```python
from build123d import *

# Parameters (mm, degrees)
BROCA_DE_ROSQUEAR_PARA_TARRAXA_DE_M51_D     = 4.2
BROCA_DE_ROSQUEAR_PARA_TARRAXA_DE_M51_DEPTH = 10
BROCA_DE_ROSQUEAR_PARA_TARRAXA_DE_M51_TIP   = 1.2618073
CORTE_EXTRUS_O1_DEPTH                       = 69.373971656
CORTE_EXTRUS_O1_DEPTH_BACK                  = 69.373971656
ESBO_O8_W                                   = 1
ESBO_O8_H                                   = 4


with BuildPart() as part:
    # Esboço1 → Revolução1 (revolve)
    with BuildSketch(Plane.XY, mode=Mode.PRIVATE) as revolu_o1_sk:
        Polygon((0, 0), (-5, 0), (-5, 60), (-15, 60), (-15, 65), (0, 65), align=None)
    revolve(revolu_o1_sk.sketch.rotate(Axis((0, 0, 0), (0, 1, 0)), 270), axis=Axis((0, 0, 0), (0, 1, 0)))

    # Broca de rosquear para tarraxa de M51
    with Locations(Plane(origin=(0, 0, 0), x_dir=(-1, 0, 0), z_dir=(0, -1, 0))):
        with Locations((0, 0)):
            Hole(BROCA_DE_ROSQUEAR_PARA_TARRAXA_DE_M51_D / 2, depth=BROCA_DE_ROSQUEAR_PARA_TARRAXA_DE_M51_DEPTH)
            with Locations((0, 0, -(BROCA_DE_ROSQUEAR_PARA_TARRAXA_DE_M51_DEPTH + BROCA_DE_ROSQUEAR_PARA_TARRAXA_DE_M51_TIP / 2))):  # 118° drill point
                Cone(0, BROCA_DE_ROSQUEAR_PARA_TARRAXA_DE_M51_D / 2, BROCA_DE_ROSQUEAR_PARA_TARRAXA_DE_M51_TIP, mode=Mode.SUBTRACT)

    # Esboço8 → Corte-extrusão1 (cut, two sides: drawn at the far end of the back side and taken through both)
    with BuildSketch(Plane.XY.offset(-CORTE_EXTRUS_O1_DEPTH_BACK)):
        with Locations((4.5, 2)):
            Rectangle(ESBO_O8_W, ESBO_O8_H)
        with Locations((-4.5, 2)):
            Rectangle(ESBO_O8_W, ESBO_O8_H)
    extrude(amount=CORTE_EXTRUS_O1_DEPTH + CORTE_EXTRUS_O1_DEPTH_BACK, mode=Mode.SUBTRACT)


solid = part.part
```
Check sheet for the modelled part. Datum: model origin and axes. Units: mm. A direction names the side the tool comes from. Round coordinates to 2 decimals unless told otherwise and drop trailing zeros. Loops run counter-clockwise (first coordinate to the right, second up) from the corner with the lowest first, then second, coordinate; pieces in that order, holes last. Notation, with made-up numbers: (87.5, 78.5) -> (92.5, 78.5) arc R16 ccw to (92.5, 98.5) -> close; hole circle Ø8 at (2, 38.5). An arc over 180 degrees is marked (long way). Answer in a Markdown table with one row per item.
Q1. Sectioned sample at D-D on y = 40.5. Enter the section's corners in (x, z), then the cut area to 3 significant figures.
Data:
| item | result |
|---|---|
| outline | circle Ø10 at (0, 0) |
| area | 78.5 mm^2 |
Q2. Set-up check for faces 4 (the face through (-4, 2, 0)), 5 (the face through (-0.1, 0, -2.3)), 6 (the face through (0, 30, 5)): record each of +Z, -Z, +X, -X, +Y, -Y from which the full face is reachable in a straight line by a thin tool's end or side.
Data:
| item | result |
|---|---|
| face 4 | +Z, -Z, -X, -Y |
| face 5 | +Z, -Z, +X, -X, -Y |
| face 6 | -Y |
Q3. Release check for a two-part mould opening along X. For faces 1 (the face through (2.003, 5.07, -0.631)), 2 (the face through (4, 2, 0)), 3 (the face through (-4, 60, -4)) record: released by +X, released by -X, zero draft, split by the parting line, or undercut.
Data:
| item | result |
|---|---|
| face 1 | undercut |
| face 2 | released by +X |
| face 3 | zero draft |
Q4. Go/stop test with flat-tipped pins: P1, Ø1, axis at y = 10, z = 3.5, coming from the +X side; P2, Ø6, axis at y = 9.5, z = 4.5, coming from the +X side; P3, Ø2, axis at y = 1, z = 0, coming from the -X side. Record where each tip stops, or that it passes through.
Data:
| item | result |
|---|---|
| P1 | stops at x = 4 |
| P2 | stops at x = 4.77 |
| P3 | stops at x = -4 |
Q5. Sectioned sample at B-B on x = -11.5. Enter the section's corners in (y, z), then the cut area to 3 significant figures.
Data:
| item | result |
|---|---|
| outline | (60, -9.63) -> (65, -9.63) -> (65, 9.63) -> (60, 9.63) -> close |
| area | 96.3 mm^2 |
Q6. Sectioned sample at A-A on y = 5.5. Enter the section's corners in (x, z).
Data:
| item | result |
|---|---|
| outline | circle Ø10 at (0, 0); hole circle Ø4.2 at (0, 0) |
Q7. Sectioned sample at C-C on z = 13. Enter the section's corners in (x, y).
Data:
| item | result |
|---|---|
| outline | (-7.48, 60) -> (7.48, 60) -> (7.48, 65) -> (-7.48, 65) -> close |
Q8. Thickness scan on L1, parallel to Y at x = 8.5, z = 0.75; L2, parallel to X at y = 16.5, z = -2.75; L3, parallel to Z at x = 4.25, y = 23. Record the ranges inside material, lowest first.
Data:
| item | result |
|---|---|
| L1 | y = 60 to 65 |
| L2 | x = -4.18 to 4.18 |
| L3 | z = -2.63 to 2.63 |
